Read the model definition and answer for the solid it produces. Units are mm, in the model's axes. Face numbers are marked on the shaded views. A direction names the side the tool comes from. Coordinates: 2 decimals unless noted, no trailing zeros. Order: outer loops, then holes, each group sorted by start corner. A loop starts at its lowest first (then second) coordinate and runs counter-clockwise, first axis right, second up. Notation, with made-up numbers: (61, -17) -> (95, -17) arc R25 cw to (95, 18) -> close; hole circle Ø3 at (34, -22). An arc over 180 degrees is marked (long way). Answer in a Markdown table with one row per item.
from build123d import *

# Parameters (mm, degrees)
SKETCH1_W           = 88.9
SKETCH1_H           = 101.6
SKETCH1_R           = 1.5
BOSS_EXTRUDE1_DEPTH = 1.5
SKETCH3_W           = 12.406
SKETCH3_H           = 16
SKETCH3_W_2         = 3.594
BOSS_EXTRUDE2_DEPTH = 15
SKETCH3_3_W         = 12.16
SKETCH3_3_H         = 12
SKETCH3_3_W_2       = 3.84
BOSS_EXTRUDE3_DEPTH = 11
SKETCH3_4_W         = 12.16
SKETCH3_4_H         = 12.1
BOSS_EXTRUDE4_DEPTH = 1.5


with BuildPart() as part:
    # Sketch1 → Boss-Extrude1 (new body)
    with BuildSketch(Plane(origin=(0, 0, 0), x_dir=(1, 0, 0), z_dir=(0, 1, 0))):
        Rectangle(SKETCH1_W, SKETCH1_H)
        with Locations(Location((25.4, -44.45, 0), (0, 0, 270))):
            Circle(SKETCH1_R, mode=Mode.SUBTRACT)
        with Locations(Location((-38.1, -44.45, 0), (0, 0, 270))):
            Circle(SKETCH1_R, mode=Mode.SUBTRACT)
        with Locations(Location((25.4, 44.45, 0), (0, 0, 270))):
            Circle(SKETCH1_R, mode=Mode.SUBTRACT)
        with Locations(Location((-38.1, 44.45, 0), (0, 0, 270))):
            Circle(SKETCH1_R, mode=Mode.SUBTRACT)
    extrude(amount=BOSS_EXTRUDE1_DEPTH)

    # Sketch3 → Boss-Extrude2 (add)
    with BuildSketch(Plane(origin=(0, 1.5, 0), x_dir=(1, 0, 0), z_dir=(0, 1, 0))):
        with Locations((-38.247, 25.4)):
            Rectangle(SKETCH3_W, SKETCH3_H)
        with Locations((-46.247, 25.4)):
            Rectangle(SKETCH3_W_2, SKETCH3_H)
    extrude(amount=BOSS_EXTRUDE2_DEPTH)

    # Sketch3_3 → Boss-Extrude3 (add)
    with BuildSketch(Plane(origin=(0, 1.5, 0), x_dir=(1, 0, 0), z_dir=(0, 1, 0))):
        with Locations((-38.37, 0)):
            Rectangle(SKETCH3_3_W, SKETCH3_3_H)
        with Locations((-46.37, 0)):
            Rectangle(SKETCH3_3_W_2, SKETCH3_3_H)
    extrude(amount=BOSS_EXTRUDE3_DEPTH)

    # Sketch3_4 → Boss-Extrude4 (add)
    with BuildSketch(Plane(origin=(0, 1.5, 0), x_dir=(1, 0, 0), z_dir=(0, 1, 0))):
        with Locations((-38.37, -25.4)):
            Rectangle(SKETCH3_4_W, SKETCH3_4_H)
    extrude(amount=BOSS_EXTRUDE4_DEPTH)


solid = part.part
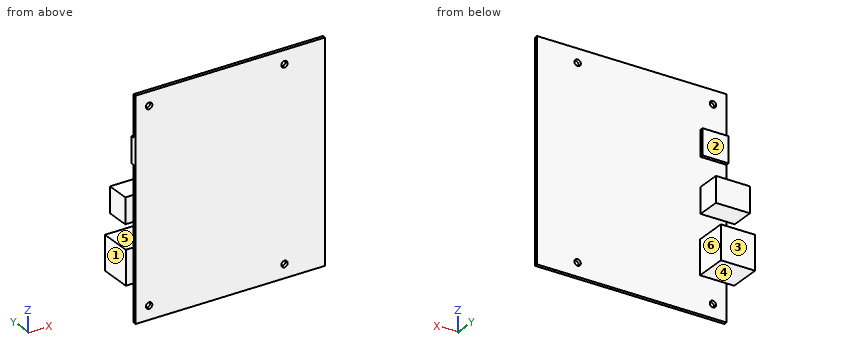
Q1. Given pin 1 (5.5 mm diameter, centred on x = -42.5, y = 9, fed in from +Z); pin 2 (9 mm diameter, centred on y = 9, z = 2.5, fed in from +X); pin 3 (2 mm diameter, centred on x = 22, y = 4, fed in from -Z); pin 4 (13 mm diameter, centred on x = -43, z = -2.5, fed in from +Y), each flat-ended and moving along its own axis, determine where each tip first touches the part or whether it passes through.
Outcome:
| item | result |
|---|---|
| pin 1 | z = 6 |
| pin 2 | x = -32.29 |
| pin 3 | through |
| pin 4 | y = 12.5 |
Q2. The part is cut by section A-A (z = -44.45). Write down the section's boundary in (x, y), then the cut area to 3 significant figures.
Outcome:
| item | result |
|---|---|
| outline | (-44.45, 0) -> (-39.6, 0) -> (-39.6, 1.5) -> (-44.45, 1.5) -> close; (-36.6, 0) -> (23.9, 0) -> (23.9, 1.5) -> (-36.6, 1.5) -> close; (26.9, 0) -> (44.45, 0) -> (44.45, 1.5) -> (26.9, 1.5) -> close |
| area | 124 mm² |
Q3. For a pull along Z with two mould halves and no side action, classify the marked faces 4, 5 and 6 as pulls with the +Z half, pulls with the -Z half, needs draft (parallel to the pull), parting line crosses it, or undercut.
Outcome:
| item | result |
|---|---|
| face 4 | pulls with the -Z half |
| face 5 | undercut |
| face 6 | needs draft |
Q4. For the marked faces 1, 2 and 3, determine the directions among +Z, -Z, +X, -X, +Y, -Y from which every point of the face is accessible in a straight line to the end or side of a thin tool.
Outcome:
| item | result |
|---|---|
| face 1 | -Z, -X, +Y, -Y |
| face 2 | +Z, +X, -X, +Y |
| face 3 | +Z, -Z, +X, -X, +Y |
Q5. The part is cut by section C-C (z = 23.5). Write down the section's boundary in (x, y), then the cut area to 3 significant figures.
Outcome:
| item | result |
|---|---|
| outline | (-44.45, 0) -> (44.45, 0) -> (44.45, 1.5) -> (-32.29, 1.5) -> (-32.29, 3) -> (-44.45, 3) -> close |
| area | 152 mm² |
Q6. The part is cut by section D-D (y = 15). Write down the section's boundary in (x, z).
Outcome:
| item | result |
|---|---|
| outline | (-48.04, -33.4) -> (-32.04, -33.4) -> (-32.04, -17.4) -> (-48.04, -17.4) -> close |
Q7. Consider line 1 (X direction, y = 1.15, z = 44.45); line 2 (Z direction, x = -37.5, y = 8.5); line 3 (Y direction, x = 32, z = 21). Determine where each line is inside the solid, lowest interval first.
Outcome:
| item | result |
|---|---|
| line 1 | -44.45 to -39.6, -36.6 to 23.9, 26.9 to 44.45 |
| line 2 | -33.4 to -17.4, -6 to 6 |
| line 3 | 0 to 1.5 |
Q8. The part is cut by section B-B (x = -38.1). Write down the section's boundary in (y, z).
Outcome:
| item | result |
|---|---|
| outline | (0, -50.8) -> (1.5, -50.8) -> (1.5, -45.95) -> (0, -45.95) -> close; (0, -42.95) -> (1.5, -42.95) -> (1.5, -33.4) -> (16.5, -33.4) -> (16.5, -17.4) -> (1.5, -17.4) -> (1.5, -6) -> (12.5, -6) -> (12.5, 6) -> (1.5, 6) -> (1.5, 19.35) -> (3, 19.35) -> (3, 31.45) -> (1.5, 31.45) -> (1.5, 42.95) -> (0, 42.95) -> close; (0, 45.95) -> (1.5, 45.95) -> (1.5, 50.8) -> (0, 50.8) -> close |
